from build123d import *

# Parameters (mm, degrees)
F0_W     = 20
F0_H     = 60
F1_DEPTH = 300
F2_W     = 20
F2_H     = 40
F3_DEPTH = 10
F4_W     = 20
F4_H     = 40
F5_DEPTH = 10


with BuildPart() as f1:
    # F0 (on Right) → F1 (new body)
    with BuildSketch(Plane.YZ):
        with Locations((10, -30)):
            Rectangle(F0_W, F0_H)
    extrude(amount=F1_DEPTH)

    # F2 (on face) → F3 (join)
    with BuildSketch(Plane(origin=(0, 0, 0), x_dir=(0, -1, 0), z_dir=(-1, 0, 0))):
        with Locations((-10, -30)):
            Rectangle(F2_W, F2_H)
    extrude(amount=F3_DEPTH)

    # F4 (on face) → F5 (join)
    with BuildSketch(Plane.YZ.offset(300)):
        with Locations((10, -30)):
            Rectangle(F4_W, F4_H)
    extrude(amount=F5_DEPTH)


solid = f1.part
The model under review builds one solid part; all positions refer to its coordinate system, in mm. A direction names the side the tool comes from. Give positions to 0.01 mm unless a question says otherwise; leave off trailing zeros. Loops run counter-clockwise (first coordinate to the right, second up) from the corner with the lowest first, then second, coordinate; pieces in that order, holes last. Notation, with made-up numbers: (20, 55) -> (31, 55) arc R24 ccw to (31, 69) -> close; hole circle Ø3 at (63, 50.25). An arc over 180 degrees is marked (long way). Answer as a JSON object with one key per item and string values. Group by question number.
Q1. Tool access review of faces 1 (the flat face through (0, 10, -55)), 2 (the flat face through (-10, 10, -30)), 3 (the flat face through (300, 10, -55)), 4 (the flat face through (-5, 10, -10)), 5 (the flat face through (305, 10, -10)): name each direction out of +Z, -Z, +X, -X, +Y, -Y from which nothing blocks a thin tool from reaching the whole face with its end or side.
Q2. Take a section at A-A (y = 16). Write out the cut boundary in (x, z), plus the area to 3 significant figures.
Q3. Insertion check: pin 1 (8 mm diameter, centred on y = 10, z = -56.5, fed in from +X); pin 2 (11 mm diameter, centred on y = 14, z = -57, fed in from -X); pin 3 (3 mm diameter, centred on x = -3.5, y = 14, fed in from -Z). Each pin has a flat end and moves straight along its axis. Give the tip position at first contact, or say it passes through.
Q4. Wall thickness on line 1 along X through (y, z) = (9.25, -9.5): over which ranges is the line inside the solid? List them lowest first.
Q5. Take a section at B-B (z = -5.5). Write out the cut boundary in (x, y).
Answer below:
{
 "1": {"face 1": "-Z, -X, +Y, -Y", "face 2": "+Z, -Z, -X, +Y, -Y", "face 3": "-Z, +X, +Y, -Y", "face 4": "+Z, -X, +Y, -Y", "face 5": "+Z, +X, +Y, -Y"},
 "2": {"outline": "(-10, -50) -> (0, -50) -> (0, -60) -> (300, -60) -> (300, -50) -> (310, -50) -> (310, -10) -> (300, -10) -> (300, 0) -> (0, 0) -> (0, -10) -> (-10, -10) -> close", "area": "18,800 mm2"},
 "3": {"pin 1": "stops at x = 300", "pin 2": "stops at x = 0", "pin 3": "stops at z = -50"},
 "4": {"line 1": "x = 0 to 300"},
 "5": {"outline": "(0, 0) -> (300, 0) -> (300, 20) -> (0, 20) -> close"}
}
